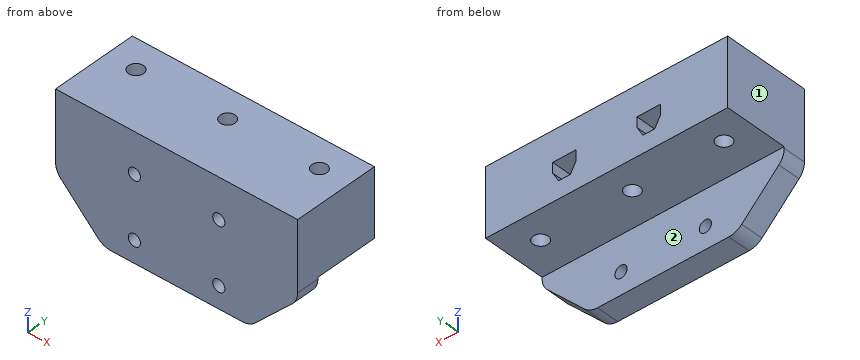
```python
from build123d import *

# Parameters (mm, degrees)
SKETCH1_W           = 62
SKETCH1_H           = 31.1
SKETCH1_R           = 3.3235
BOSS_EXTRUDE1_DEPTH = 12.446
SKETCH1_3_W         = 35
SKETCH1_3_H         = 36.9
SKETCH1_3_W_2       = 62
BOSS_EXTRUDE2_DEPTH = 47.3
SKETCH1_4_R         = 3.3235
BOSS_EXTRUDE3_DEPTH = 21
SKETCH2_R           = 4.1
CUT_EXTRUDE1_DEPTH  = 36.9
CHAMFER1_SIZE       = 40
FILLET3_R           = 10


with BuildPart() as part:
    # Sketch1 → Boss-Extrude1 (new body)
    with BuildSketch(Plane(origin=(0, 0, 0), x_dir=(1, 0, 0), z_dir=(0, 1, 0))):
        with Locations((31, -15.55)):
            Rectangle(SKETCH1_W, SKETCH1_H)
        with Locations(Location((8, -12, 0), (0, 0, 270))):
            Circle(SKETCH1_R, mode=Mode.SUBTRACT)
        with Locations(Location((54, -12, 0), (0, 0, 270))):
            Circle(SKETCH1_R, mode=Mode.SUBTRACT)
    extrude(amount=BOSS_EXTRUDE1_DEPTH)

    # Sketch1<3> → Boss-Extrude2 (add)
    # profile 1 of 3: a face of its own
    with BuildSketch(Plane(origin=(0, 0, 0), x_dir=(1, 0, 0), z_dir=(0, 1, 0))):
        with Locations((-17.5, -49.55)):
            Rectangle(SKETCH1_3_W, SKETCH1_3_H)
    # profile 2 of 3: a face of its own
    with BuildSketch(Plane(origin=(0, 0, 0), x_dir=(1, 0, 0), z_dir=(0, 1, 0))):
        with Locations((31, -49.55)):
            Rectangle(SKETCH1_3_W_2, SKETCH1_3_H)
        Polygon((1.585638509, -46), (4.792819255, -40.445), (11.207180745, -40.445), (14.414361491, -46), (14.414361491, -51.555), (11.207180745, -51.555), (4.792819255, -51.555), (1.585638509, -51.555), align=None, mode=Mode.SUBTRACT)
        Polygon((60.414361491, -46), (60.414361491, -51.555), (47.585638509, -51.555), (47.585638509, -46), (50.792819255, -40.445), (57.207180745, -40.445), align=None, mode=Mode.SUBTRACT)
    # profile 3 of 3: a face of its own
    with BuildSketch(Plane(origin=(0, 0, 0), x_dir=(1, 0, 0), z_dir=(0, 1, 0))):
        with Locations((79.5, -49.55)):
            Rectangle(SKETCH1_3_W, SKETCH1_3_H)
    extrude(amount=BOSS_EXTRUDE2_DEPTH)

    # Sketch1<4> → Boss-Extrude3 (add)
    # profile 1 of 2: a face of its own
    with BuildSketch(Plane(origin=(0, 0, 0), x_dir=(1, 0, 0), z_dir=(0, 1, 0))):
        Polygon((14.414361491, -46), (11.207180745, -40.445), (4.792819255, -40.445), (1.585638509, -46), (1.585638509, -51.555), (14.414361491, -51.555), align=None)
        with Locations(Location((8, -46, 0), (0, 0, 90))):
            Circle(SKETCH1_4_R, mode=Mode.SUBTRACT)
    # profile 2 of 2: a face of its own
    with BuildSketch(Plane(origin=(0, 0, 0), x_dir=(1, 0, 0), z_dir=(0, 1, 0))):
        Polygon((47.585638509, -51.555), (60.414361491, -51.555), (60.414361491, -46), (57.207180745, -40.445), (50.792819255, -40.445), (47.585638509, -46), align=None)
        with Locations(Location((54, -46, 0), (0, 0, 90))):
            Circle(SKETCH1_4_R, mode=Mode.SUBTRACT)
    extrude(amount=BOSS_EXTRUDE3_DEPTH)

    # Sketch2 → Cut-Extrude1 (cut)
    with BuildSketch(Plane(origin=(0, 0, 68), x_dir=(-1, 0, 0), z_dir=(0, 0, -1))):
        with Locations(Location((19, 31.47, 0), (0, 0, 180))):
            Circle(SKETCH2_R)
        with Locations(Location((-31, 31.47, 0), (0, 0, 180))):
            Circle(SKETCH2_R)
        with Locations(Location((-81, 31.47, 0), (0, 0, 180))):
            Circle(SKETCH2_R)
    extrude(amount=CUT_EXTRUDE1_DEPTH, mode=Mode.SUBTRACT)

    # Chamfer1
    # the kernel refuses this chamfer: 40 mm, written as the material it adds along each edge
    with BuildSketch(Plane(origin=(62, 0, 31.1), x_dir=(0.9996219169112968, 0, 0.02749587661058649), z_dir=(0, 1, 0))) as chamfer1_piece_1_section:
        Polygon((CHAMFER1_SIZE * 0.999621916911, CHAMFER1_SIZE * 0.0274958766106), (-CHAMFER1_SIZE * 0.0274958766106, CHAMFER1_SIZE * 0.999621916911), (0, 0), align=None)
    chamfer1_piece_1 = extrude(amount=12.446, mode=Mode.PRIVATE)
    chamfer1_piece_1 = split(chamfer1_piece_1, bisect_by=Plane(origin=(97, 6.223, 19.019433431), z_dir=(-1, 0, 0)), keep=Keep.TOP, mode=Mode.PRIVATE)
    chamfer1_piece_1 = split(chamfer1_piece_1, bisect_by=Plane(origin=(75.290949727, 6.223, 0), z_dir=(0, 0, 1)), keep=Keep.TOP, mode=Mode.PRIVATE)
    add(chamfer1_piece_1)
    with BuildSketch(Plane(origin=(0, 0, 31.1), x_dir=(-0.9996219169112968, 0, 0.027495876610586497), z_dir=(0, 1, 0))) as chamfer1_piece_2_section:
        Polygon((CHAMFER1_SIZE * 0.999621916911, -CHAMFER1_SIZE * 0.0274958766106), (-CHAMFER1_SIZE * 0.0274958766106, -CHAMFER1_SIZE * 0.999621916911), (0, 0), align=None)
    chamfer1_piece_2 = extrude(amount=12.446, mode=Mode.PRIVATE)
    chamfer1_piece_2 = split(chamfer1_piece_2, bisect_by=Plane(origin=(-35, 6.223, 19.019433431), z_dir=(1, 0, 0)), keep=Keep.TOP, mode=Mode.PRIVATE)
    chamfer1_piece_2 = split(chamfer1_piece_2, bisect_by=Plane(origin=(-13.290949727, 6.223, 0), z_dir=(0, 0, 1)), keep=Keep.TOP, mode=Mode.PRIVATE)
    add(chamfer1_piece_2)

    # Fillet3
    fillet3_edges = [part.edges().sort_by_distance(p)[0] for p in [
        (70.9, 6.223, 0),
        (97, 6.223, 26.1),
        (-35, 6.223, 26.1),
        (-8.9, 6.223, 0),
    ]]
    fillet(fillet3_edges, radius=FILLET3_R)


solid = part.part
```
CAD build for the part. Positions are in the model's coordinates, mm. Face numbers are marked on the shaded views. A direction names the side the tool comes from. Round coordinates to 2 decimals unless told otherwise and drop trailing zeros. Loops run counter-clockwise (first coordinate to the right, second up) from the corner with the lowest first, then second, coordinate; pieces in that order, holes last. Notation, with made-up numbers: M 50.25,38 L 54.25,38 A27 cw 54.25,74 Z; hole C -13.5,22 d3. An arc over 180 degrees is marked long. Return JSON: item names as keys, results as strings. Group by question number.
(1) Saw through at B-B, the plane y = 31.47. List the corners of the cut face in (x, z) (3 decimals).
(2) Saw through at C-C, the plane z = 55.5. List the corners of the cut face in (x, y).
(3) Saw through at A-A, the plane x = 31. List the corners of the cut face in (y, z), and give its area (3 significant figures).
(4) Drop flat-ended pins along their axis: P1, Ø3, axis at y = 29.5, z = 29.5, coming from the -X side; P2, Ø7.5, axis at x = 54, z = 12, coming from the +Y side; P3, Ø9.5, axis at x = -19, y = 31.47, coming from the +Z side; P4, Ø10.5, axis at x = 8, z = 46, coming from the +Y side. Give the stop position or say it passes through.
(5) Saw through at D-D, the plane x = 8. List the corners of the cut face in (y, z) (1 decimal), and give its area (3 significant figures).
(6) Tool access for the marked faces 1 and 2: list every direction of +Z, -Z, +X, -X, +Y, -Y with a clear straight run to the whole face (end or side of a thin tool).
(7) Wall check: probe 1 along X at (y, z) = (43, 49); probe 2 along X at (y, z) = (16.5, 46); probe 3 along Z at (x, y) = (8, 16.25). Give the ranges that are in metal, low to high. Write a range as [from, to].
Answer list:
{
 "1": {"outline": "M -35,31.1 L -23.1,31.1 L -23.1,68 L -35,68 Z; M -14.9,31.1 L 26.9,31.1 L 26.9,68 L -14.9,68 Z; M 35.1,31.1 L 76.9,31.1 L 76.9,68 L 35.1,68 Z; M 85.1,31.1 L 97,31.1 L 97,68 L 85.1,68 Z; hole M 1.586,46 L 4.793,40.445 L 11.207,40.445 L 14.414,46 L 14.414,51.555 L 1.586,51.555 Z; hole M 47.586,46 L 50.793,40.445 L 57.207,40.445 L 60.414,46 L 60.414,51.555 L 47.586,51.555 Z"},
 "2": {"outline": "M -35,0 L 97,0 L 97,47.3 L -35,47.3 Z; hole C -19,31.47 d8.2; hole C 31,31.47 d8.2; hole C 81,31.47 d8.2"},
 "3": {"outline": "M 0,0 L 12.45,0 L 12.45,31.1 L 27.37,31.1 L 27.37,68 L 0,68 Z; M 35.57,31.1 L 47.3,31.1 L 47.3,68 L 35.57,68 Z", "area": "1,830 mm2"},
 "4": {"P1": "through", "P2": "y = 12.45", "P3": "z = 68", "P4": "y = 21"},
 "5": {"outline": "M 0,0 L 12.4,0 L 12.4,8.7 L 0,8.7 Z; M 0,15.3 L 12.4,15.3 L 12.4,31.1 L 47.3,31.1 L 47.3,40.4 L 21,40.4 L 21,42.7 L 0,42.7 Z; M 0,49.3 L 21,49.3 L 21,51.6 L 47.3,51.6 L 47.3,68 L 0,68 Z", "area": "1,620 mm2"},
 "6": {"face 1": "+Z, -Z, -X, +Y, -Y", "face 2": "-Z, +X, -X, +Y"},
 "7": {"probe 1": "[-35, 1.59], [14.41, 47.59], [60.41, 97]", "probe 2": "[-35, 4.68], [11.32, 50.68], [57.32, 97]", "probe 3": "[31.1, 42.68], [49.32, 68]"}
}
